Check sheet for the modelled part. Datum: model origin and axes. Units: mm. Face numbers are marked on the shaded views. A direction names the side the tool comes from. Round coordinates to 2 decimals unless told otherwise and drop trailing zeros. Loops run counter-clockwise (first coordinate to the right, second up) from the corner with the lowest first, then second, coordinate; pieces in that order, holes last. Notation, with made-up numbers: (26, 16) - (34, 16) arc R18 cw to (34, 45) - close; hole circle Ø3 at (40, -35.75). An arc over 180 degrees is marked (long way). Return JSON: item names as keys, results as strings.
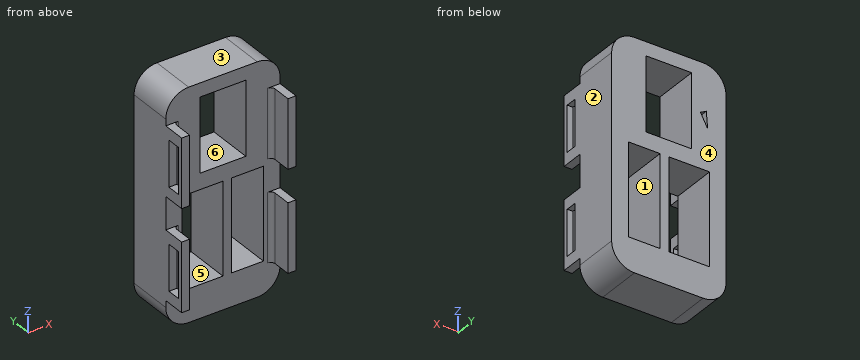
Autodesk Inventor part; units mm, degrees
ref_plane "YZ Plane" through (0, 0, 0) normal (1, 0, 0) x (0, 1, 0)
ref_plane "XZ Plane" through (0, 0, 0) normal (0, 1, 0) x (-1, 0, 0)
ref_plane "XY Plane" through (0, 0, 0) normal (0, 0, 1) x (1, 0, 0)
sketch "Sketch1" plane through (0, 0, 0) normal (0, 1, 0) x (-1, 0, 0)
  line L0 (29.9672, 50.4505) -> (-0.0328, 50.4505)
  line L1 (-10.0328, 40.4505) -> (-10.0328, -39.5495)
  line L2 (-0.0328, -49.5495) -> (29.9672, -49.5495)
  line L3 (39.9672, -39.5495) -> (39.9672, 40.4505)
  line L4 (24.9672, 44.4505) -> (4.9672, 44.4505)
  line L5 (4.9672, 44.4505) -> (4.9672, 12.105)
  line L6 (4.9672, 12.105) -> (24.9672, 12.105)
  line L7 (24.9672, 12.105) -> (24.9672, 44.4505)
  line L8 (32.8329, 5.1351) -> (14.9672, 5.1351)
  line L9 (14.9672, 5.1351) -> (14.9672, -35.2063)
  line L10 (14.9672, -35.2063) -> (32.8329, -35.2063)
  line L11 (32.8329, -35.2063) -> (32.8329, 5.1351)
  line L12 (11.1837, 5.1351) -> (-2.7562, 5.1351)
  line L13 (-2.7562, 5.1351) -> (-2.7562, -35.2063)
  line L14 (-2.7562, -35.2063) -> (11.1837, -35.2063)
  line L15 (11.1837, -35.2063) -> (11.1837, 5.1351)
  arc A0 (-0.0328, 50.4505) -> (-10.0328, 40.4505) centre (-0.0328, 40.4505) ccw
  arc A1 (39.9672, 40.4505) -> (29.9672, 50.4505) centre (29.9672, 40.4505) ccw
  arc A2 (29.9672, -49.5495) -> (39.9672, -39.5495) centre (29.9672, -39.5495) ccw
  arc A3 (-10.0328, -39.5495) -> (-0.0328, -49.5495) centre (-0.0328, -39.5495) ccw
  point P0 (0, 0)
  point P1 (39.9672, 50.4505)
  point P2 (-10.0328, -49.5495)
  point P3 (39.9672, -49.5495)
  dimension "d1" = 100
  dimension "d2" = 50
  dimension "d3" = 15
  dimension "d4" = 15
  dimension "d6" = 6
  dimension "d7" = 10
  dimension "d8" = 10
  dimension "d9" = 10
  dimension "d10" = 10
extrude "Extrusion1" add sketch "Sketch1" along normal blind 20
sketch "Sketch2" plane through (0, 0, 0) normal (0, -1, 0) x (1, 0, 0)
  line L0 (10.0328, 40.4505) -> (10.0328, -39.5495)
  line L1 (10.0328, 37.5913) -> (6.5328, 37.5913)
  line L2 (6.5328, 37.5913) -> (6.5328, 7.5913)
  line L3 (6.5328, 7.5913) -> (10.0328, 7.5913)
  line L4 (10.0328, 7.5913) -> (10.0328, 37.5913)
  line L5 (10.0328, -6.6206) -> (6.5328, -6.6206)
  line L6 (6.5328, -6.6206) -> (6.5328, -36.6206)
  line L7 (6.5328, -36.6206) -> (10.0328, -36.6206)
  line L8 (10.0328, -36.6206) -> (10.0328, -6.6206)
  arc A0 (10.0328, 40.4505) -> (0.0328, 50.4505) centre (0.0328, 40.4505) ccw
  arc A1 (0.0328, -49.5495) -> (10.0328, -39.5495) centre (0.0328, -39.5495) ccw
  line L9 (-39.9672, -39.5495) -> (-39.9672, 40.4505)
  line L10 (-39.9672, 37.5913) -> (-36.4672, 37.5913)
  line L11 (-36.4672, 37.5913) -> (-36.4672, 7.5913)
  line L12 (-36.4672, 7.5913) -> (-39.9672, 7.5913)
  line L13 (-39.9672, 7.5913) -> (-39.9672, 37.5913)
  line L14 (-39.9672, -6.6206) -> (-36.4672, -6.6206)
  line L15 (-36.4672, -6.6206) -> (-36.4672, -36.6206)
  line L16 (-36.4672, -36.6206) -> (-39.9672, -36.6206)
  line L17 (-39.9672, -36.6206) -> (-39.9672, -6.6206)
  point P0 (0, 0)
  point P1 (7.1038, 47.5215)
  point P2 (8.2828, 37.5913)
  point P3 (7.1038, -46.6206)
  point P4 (8.2828, 7.5913)
  point P5 (-34.5818, 22.0482)
  point P6 (-38.0818, -7.9518)
  point P7 (-37.5107, 76.1904)
  point P8 (-36.4672, -21.6206)
  point P9 (-39.9672, -21.6206)
  dimension "d13" = 3.5
  dimension "d14" = 3.5
  dimension "d15" = 10
  dimension "d16" = 10
  dimension "d17" = 30
  dimension "d18" = 30
  dimension "d22" = 3.5
  dimension "d23" = 3.5
extrude "Extrusion2" add sketch "Sketch2" along normal blind 10
fillet "Fillet1" radius 2 4 edges at (6.5328, 0, 22.5913) (6.5328, 0, -21.6206) (-36.4672, 0, 22.5913) (-36.4672, 0, -21.6206)
sketch "Sketch3" plane through (10.0328, 0, -39.5495) normal (1, 0, 0) x (0, 0, -1)
  line L0 (-72.1408, -3) -> (-52.1157, -3)
  line L1 (-52.1157, -3) -> (-52.1157, -8)
  line L2 (-52.1157, -8) -> (-72.1408, -8)
  line L3 (-72.1408, -8) -> (-72.1408, -3)
  line L4 (-77.1408, 0) -> (-77.1408, -10)
  line L5 (-47.1408, 0) -> (-47.1408, -10)
  line L6 (-77.1408, 0) -> (-47.1408, 0)
  line L7 (-27.9289, -3) -> (-7.9289, -3)
  line L8 (-7.9289, -3) -> (-7.9289, -8)
  line L9 (-7.9289, -8) -> (-27.9289, -8)
  line L10 (-27.9289, -8) -> (-27.9289, -3)
  line L11 (-32.9289, 0) -> (-32.9289, -10)
  line L12 (-2.9289, 0) -> (-2.9289, -10)
  point P0 (-39.5495, 0)
  point P1 (-77.1408, -5)
  point P2 (-52.1157, -5.5)
  point P3 (-47.1408, -5)
  point P4 (-32.9289, -5)
  point P5 (-27.9289, -5.5)
  point P6 (-2.9289, -5)
  point P7 (-7.9289, -5.5)
  dimension "d27" = 5
  dimension "d28" = 5
  dimension "d29" = 5
  dimension "d30" = 3
  dimension "d31" = 5
  dimension "d33" = 5
extrude "Extrusion3" cut sketch "Sketch3" against normal blind 2.5
sketch "Sketch4" plane through (0, 20, 0) normal (0, 1, 0) x (1, 0, 0)
  point P0 (0, 0)
sketch "Sketch5" plane through (0, 20, 0) normal (0, 1, 0) x (1, 0, 0)
  line L0 (-31.3896, -30.3859) -> (-31.9666, -23.1707)
  line L1 (-31.9666, -23.1707) -> (-28.8346, -29.0171)
  line L2 (-28.8346, -29.0171) -> (-31.3896, -30.3859)
  point P0 (0, 0)
extrude "Extrusion4" cut sketch "Sketch5" against normal blind 5
sketch "Sketch6" plane through (-39.9672, 0, 40.4505) normal (-1, 0, 0) x (0, 0, 1)
  line L0 (-47.0711, -2) -> (-77.0711, -2)
  line L1 (-72.0711, -2) -> (-52.0711, -2)
  line L2 (-52.0711, -2) -> (-52.0711, -8)
  line L3 (-52.0711, -8) -> (-72.0711, -8)
  line L4 (-72.0711, -8) -> (-72.0711, -2)
  line L5 (-47.0711, 0) -> (-47.0711, -10)
  line L6 (-77.0711, 0) -> (-77.0711, -10)
  line L7 (-47.0711, -10) -> (-77.0711, -10)
  line L8 (-2.8592, -2) -> (-32.8592, -2)
  line L9 (-27.8843, -8) -> (-7.8592, -8)
  line L10 (-27.8592, -2) -> (-7.8592, -2)
  line L11 (-7.8592, -2) -> (-7.8592, -8)
  line L12 (-7.8592, -8) -> (-27.8592, -8)
  line L13 (-27.8592, -8) -> (-27.8592, -2)
  line L14 (-32.8592, 0) -> (-32.8592, -10)
  point P0 (-40.4505, 0)
  point P1 (-47.0711, -5)
  point P2 (-77.0711, -5)
  point P3 (-32.8592, -5)
  point P4 (-27.8592, -5)
  point P5 (-7.8592, -2)
  dimension "d38" = 5
  dimension "d39" = 5
  dimension "d40" = 2
  dimension "d41" = 5
extrude "Extrusion5" cut sketch "Sketch6" against normal blind 5 contours L2 L3 L4 L0 | L11 L9 L13 L8
properties part number "Testing"
Q1. Sectioned sample at C-C (y = 5). Enter the section's corners in (x, z) (1 decimal).
Answer key:
{"outline": "(-40, -39.5) arc R10 ccw to (-30, -49.5) - (0, -49.5) arc R10 ccw to (10, -39.5) - (10, 40.5) arc R10 ccw to (0, 50.5) - (-30, 50.5) arc R10 ccw to (-40, 40.5) - close; hole (-32.8, -35.2) - (-15, -35.2) - (-15, 5.1) - (-32.8, 5.1) - close; hole (-25, 12.1) - (-5, 12.1) - (-5, 44.5) - (-25, 44.5) - close; hole (-11.2, -35.2) - (2.8, -35.2) - (2.8, 5.1) - (-11.2, 5.1) - close"}
Q2. Draft check along Z on the marked faces 3, 4, 5 and 6. Enter one of: released by +Z, released by -Z, zero draft, split by the parting line, or undercut.
Answer key:
{"face 3": "released by +Z", "face 4": "zero draft", "face 5": "undercut", "face 6": "undercut"}
Q3. Tool access check on the marked faces 1 and 2. Record the directions out of +Z, -Z, +X, -X, +Y, -Y that give a thin tool (end or side, any length) a straight path to the whole face; none if there is none.
Answer key:
{"face 1": "+Y, -Y", "face 2": "+Z, -Z, +X, +Y, -Y"}
Q4. Sectioned sample at B-B (x = -10). Enter the section's corners in (y, z) (1 decimal), plus the area to 3 significant figures.
Answer key:
{"outline": "(0, -49.5) - (20, -49.5) - (20, -35.2) - (0, -35.2) - close; (0, 5.1) - (20, 5.1) - (20, 12.1) - (0, 12.1) - close; (0, 44.5) - (20, 44.5) - (20, 50.5) - (0, 50.5) - close", "area": "546 mm²"}
Q5. Sectioned sample at D-D (x = -27). Enter the section's corners in (y, z).
Answer key:
{"outline": "(0, -49.55) - (20, -49.55) - (20, -35.21) - (0, -35.21) - close; (0, 5.14) - (20, 5.14) - (20, 50.45) - (0, 50.45) - close"}
Q6. Sectioned sample at A-A (z = 17). Enter the section's corners in (x, y).
Answer key:
{"outline": "(-39.97, -10) - (-36.47, -10) - (-36.47, -8) - (-39.97, -8) - close; (-39.97, -2) - (-36.47, -2) arc R2 cw to (-34.47, 0) - (-24.97, 0) - (-24.97, 20) - (-39.97, 20) - close; (-4.97, 0) - (4.53, 0) arc R2 cw to (6.53, -2) - (6.53, -10) - (10.03, -10) - (10.03, -8) - (7.53, -8) - (7.53, -3) - (10.03, -3) - (10.03, 20) - (-4.97, 20) - close"}
Q7. Depth check by flat-ended pin: P1, Ø3, axis at x = -37.5, y = -6.5, coming from the -Z side; P2, Ø1.2, axis at x = 8.5, y = -5, coming from the +Z side; P3, Ø2, axis at x = -13, z = -31.5, coming from the -Y side. Enter the tip coordinate at first touch or a pass-through.
Answer key:
{"P1": "stops at z = -36.62", "P2": "stops at z = 37.59", "P3": "stops at y = 0"}
Q8. Scan lines: probe 1 along Z at (x, y) = (-16.5, 2) (1 decimal); probe 2 along X at (y, z) = (1, -2); probe 3 along Y at (x, z) = (-36.5, -15). Record each from-to range of solid material in increasing order. Write a range as [from, to].
Answer key:
{"probe 1": "z = [-49.5, -35.2], [5.1, 12.1], [44.5, 50.5]", "probe 2": "x = [-39.97, -32.83], [-14.97, -11.18], [2.76, 10.03]", "probe 3": "y = [-10, -8], [-2, 20]"}
